```python
from build123d import *

# Parameters (mm, degrees)
F1_DEPTH = 77.216
F2_R     = 35.955946
F3_DEPTH = 87.884
F4_R     = 3.205496
F4_R_2   = 3.551228
F4_R_3   = 3.174776
F4_R_4   = 3.174773
F5_DEPTH = 95.504


with BuildPart() as f1:
    # F0 (on Top) → F1 (new body)
    with BuildSketch(Plane.XY):
        Polygon((0.305662, -58.799351), (51.074563, -29.134964), (50.768901, 29.664386), (-0.305662, 58.799351), (-51.074563, 29.134964), (-50.768901, -29.664386), align=None)
    extrude(amount=F1_DEPTH)

    # F2 (on Top) → F3 (cut)
    with BuildSketch(Plane.XY):
        Circle(F2_R)
    extrude(amount=F3_DEPTH, mode=Mode.SUBTRACT)

    # F4 (on Top) → F5 (cut)
    with BuildSketch(Plane.XY):
        with Locations((-44.734024, 0)):
            Circle(F4_R)
        with Locations((44.350594, 0)):
            Circle(F4_R_2)
        with Locations((0, 46.139952)):
            Circle(F4_R_3)
        with Locations((0, -46.012141)):
            Circle(F4_R_4)
    extrude(amount=F5_DEPTH, mode=Mode.SUBTRACT)


solid = f1.part
```
For this review, take the finished solid that the model builds, in its own axes (mm). Coordinates: 2 decimals unless noted, no trailing zeros. Loops run counter-clockwise (first coordinate to the right, second up) from the corner with the lowest first, then second, coordinate; pieces in that order, holes last. Notation, with made-up numbers: (74.25, 54) - (93.25, 54) arc R14 cw to (93.25, 68) - close; hole circle Ø1 at (-5, 85.5). An arc over 180 degrees is marked (long way). Use one line per item in the form item = value. Start each with the question number.
1) To check wall thickness, follow probe 1 along X at (y, z) = (0, 40.5); probe 2 along Y at (x, z) = (-23, 30); probe 3 along Y at (x, z) = (-46.5, 42.5). State the ranges of each line that lie inside material, in increasing order. Write a range as from..to.
2) Take a section at B-B (y = 14.5). State the section outline as (x, z) points.
3) For pin 1 (1 mm diameter, centred on x = -27.5, y = -45, fed in from +Z); pin 2 (4 mm diameter, centred on y = 24.5, z = 48.5, fed in from -X); pin 3 (1 mm diameter, centred on x = -17.5, z = 54, fed in from +Y); pin 4 (12 mm diameter, centred on y = -1.5, z = 15, fed in from +X), all flat-tipped, find the tip position at first contact; note any pin that passes through.
4) Draft analysis for pull direction Y (two halves, no side actions). For faces 1 (the face through (25.589, 44.028, 38.067)), 2 (the face through (-1, -38, 0)), 3 (the face through (47.63, -1.36, 38.07)), state which applies: released by +Y, released by -Y, zero draft, split by the parting line, or undercut.
5) Take a section at A-A (x = 25). State the section outline as (y, z) points, plus the area to 3 significant figures.
6) Take a section at D-D (y = 0). State the section outline as (x, z) points, plus the area to 3 significant figures.
7) Take a section at C-C (z = 58). State the section outline as (x, y) points, plus the area to 3 significant figures.
From the geometry:
q1.probe_1 = -50.92..-47.94, -41.53..-35.96, 35.96..40.8, 47.9..50.92
q1.probe_2 = -45.5..-27.64, 27.64..45.54
q1.probe_3 = -32.1..-2.68, 2.68..31.81
q2.outline = (-51, 0) - (-32.9, 0) - (-32.9, 77.22) - (-51, 77.22) - close; (32.9, 0) - (50.85, 0) - (50.85, 77.22) - (32.9, 77.22) - close
q3.pin_1 = through
q3.pin_2 = -51.06
q3.pin_3 = 49.04
q3.pin_4 = 50.96
q4.face_1 = released by +Y
q4.face_2 = zero draft
q4.face_3 = undercut
q5.outline = (-44.37, 0) - (-25.84, 0) - (-25.84, 77.22) - (-44.37, 77.22) - close; (25.84, 0) - (44.36, 0) - (44.36, 77.22) - (25.84, 77.22) - close
q5.area = 2,860 mm2
q6.outline = (-50.92, 0) - (-47.94, 0) - (-47.94, 77.22) - (-50.92, 77.22) - close; (-41.53, 0) - (-35.96, 0) - (-35.96, 77.22) - (-41.53, 77.22) - close; (35.96, 0) - (40.8, 0) - (40.8, 77.22) - (35.96, 77.22) - close; (47.9, 0) - (50.92, 0) - (50.92, 77.22) - (47.9, 77.22) - close
q6.area = 1,270 mm2
q7.outline = (-51.07, 29.13) - (-50.77, -29.66) - (0.31, -58.8) - (51.07, -29.13) - (50.77, 29.66) - (-0.31, 58.8) - close; hole circle Ø6.41 at (-44.73, 0); hole circle Ø71.91 at (0, 0); hole circle Ø6.35 at (0, -46.01); hole circle Ø6.35 at (0, 46.14); hole circle Ø7.1 at (44.35, 0)
q7.area = 4,790 mm2
